Check sheet for the modelled part. Datum: model origin and axes. Units: mm. Coordinates: 2 decimals unless noted, no trailing zeros. Order: outer loops, then holes, each group sorted by start corner. A loop starts at its lowest first (then second) coordinate and runs counter-clockwise, first axis right, second up.
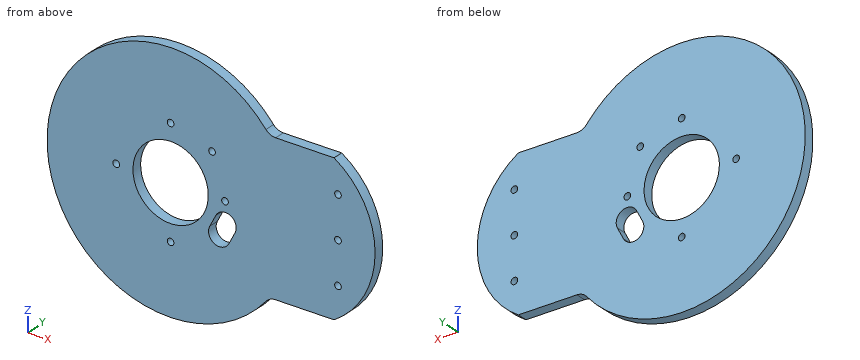
from build123d import *

# Parameters (mm, degrees)
SKETCH1_R                   = 2.0193
BOSS_EXTRUDE1_DEPTH         = 6.35
SKETCH16_R                  = 22.86
SKETCH16_R_2                = 2.0193
CUT_EXTRUDE1_DEPTH          = 6.35
FILLET1_R                   = 7.62
F_21_0_159_DIAMETER_HOLE1_D = 4.0386
CUT_EXTRUDE2_DEPTH          = 168.826775285
CUT_EXTRUDE3_DEPTH          = 168.826775285


with BuildPart() as part:
    # Sketch1 → Boss-Extrude1 (new body)
    with BuildSketch(Plane(origin=(0, 0, 0), x_dir=(1, 0, 0), z_dir=(0, 1, 0))):
        with BuildLine():
            Line((24.199172761, -44.999955873), (-14.950739381, -44.936113543))
            ThreePointArc((-14.950739381, -44.936113543), (-150.001077441, -0.07990002), (-15.0466181, 45.063954554))
            Line((-15.0466181, 45.063954554), (24.199172761, 44.999955873))
            ThreePointArc((24.199172761, 44.999955873), (71.663954553, 0), (24.199172761, -44.999955873))
        make_face()
        with Locations(Location((26.6, 0, 0), (0, 0, 270))):
            Circle(SKETCH1_R, mode=Mode.SUBTRACT)
    extrude(amount=BOSS_EXTRUDE1_DEPTH)

    # Sketch16 → Cut-Extrude1 (cut)
    with BuildSketch(Plane(origin=(0.964771866, 6.35, 105.934324836), x_dir=(-1, 0, 0), z_dir=(0, 1, 0))):
        with Locations(Location((75.964771866, -105.934324836, 0), (0, 0, 90))):
            Circle(SKETCH16_R)
        with Locations(Location((50.800979112, -80.770532082, 0), (0, 0, 90))):
            Circle(SKETCH16_R_2)
        with Locations(Location((42.944771866, -105.934324836, 0), (0, 0, 90))):
            Circle(SKETCH16_R_2)
        with Locations(Location((75.964771866, -72.914324836, 0), (0, 0, 90))):
            Circle(SKETCH16_R_2)
        with Locations(Location((108.984771866, -105.934324836, 0), (0, 0, 90))):
            Circle(SKETCH16_R_2)
        with Locations(Location((75.964771866, -138.954324836, 0), (0, 0, 90))):
            Circle(SKETCH16_R_2)
    extrude(amount=-CUT_EXTRUDE1_DEPTH, mode=Mode.SUBTRACT)

    # Fillet1
    fillet1_edges = [part.edges().sort_by_distance(p)[0] for p in [
        (-15.0466181, 3.175, -45.063954554),
        (-14.950739381, 3.175, 44.936113543),
    ]]
    fillet(fillet1_edges, radius=FILLET1_R)

    # #21 (0.159) Diameter Hole1 (through all)
    with Locations(Plane(origin=(0, 6.35, 0), x_dir=(1, 0, 0), z_dir=(0, 1, 0))):
        with Locations((26.6, 25.4), (26.6, -25.4)):
            Hole(F_21_0_159_DIAMETER_HOLE1_D / 2)

    # Sketch19 → Cut-Extrude2 (cut, through all)
    with BuildSketch(Plane(origin=(0, 6.35, 0), x_dir=(1, 0, 0), z_dir=(0, 1, 0))):
        with BuildLine():
            ThreePointArc((24.199172761, 44.999955873), (49.131977277, 0), (24.199172761, -44.999955873))
            ThreePointArc((24.199172761, -44.999955873), (71.663954553, 0), (24.199172761, 44.999955873))
        make_face()
    extrude(amount=-CUT_EXTRUDE2_DEPTH, mode=Mode.SUBTRACT)

    # Sketch20 → Cut-Extrude3 (cut, through all)
    with BuildSketch(Plane(origin=(0, 6.35, 0), x_dir=(1, 0, 0), z_dir=(0, 1, 0))):
        with BuildLine():
            Line((-39.61253295, 22.813806704), (-35.939374007, 15.716554888))
            ThreePointArc((-35.939374007, 15.716554888), (-38.746700574, 6.886169325), (-47.577086137, 9.693495892))
            Line((-47.577086137, 9.693495892), (-51.25024508, 16.790747709))
            ThreePointArc((-51.25024508, 16.790747709), (-48.442918513, 25.621133271), (-39.61253295, 22.813806704))
        make_face()
    extrude(amount=-CUT_EXTRUDE3_DEPTH, mode=Mode.SUBTRACT)


solid = part.part
(1) Cross-section at B-B (x = -75). Enter the section's corners in (y, z), and give its area (3 significant figures).
Filled in:
outline: (0, -75) - (6.35, -75) - (6.35, -35.04) - (0, -35.04) - close; (0, -31) - (6.35, -31) - (6.35, -22.86) - (0, -22.86) - close; (0, 22.86) - (6.35, 22.86) - (6.35, 31) - (0, 31) - close; (0, 35.04) - (6.35, 35.04) - (6.35, 75) - (0, 75) - close
area: 611 mm2
(2) Cross-section at C-C (y = 5). Count the separate pieces of the cut face and the enclosed holes in it, and give its area (3 significant figures).
Filled in:
separate pieces: 1
enclosed holes: 10
area: 19,900 mm2
(3) Go/stop test with flat-tipped pins: P1, Ø3, axis at x = -75, z = -33.02, coming from the -Y side; P2, Ø1.5, axis at x = 29, y = 3.5, coming from the +Z side; P3, Ø1.5, axis at x = -77, y = 4.5, coming from the +Z side. Record where each tip stops, or that it passes through.
Filled in:
P1: passes through
P2: stops at z = 42.2
P3: stops at z = 74.99
(4) Cross-section at A-A (z = 0). Enter the section's corners in (x, y).
Filled in:
outline: (-150, 0) - (-110.04, 0) - (-110.04, 6.35) - (-150, 6.35) - close; (-106, 0) - (-97.86, 0) - (-97.86, 6.35) - (-106, 6.35) - close; (-52.14, 0) - (-44, 0) - (-44, 6.35) - (-52.14, 6.35) - close; (-39.96, 0) - (24.58, 0) - (24.58, 6.35) - (-39.96, 6.35) - close; (28.62, 0) - (49.13, 0) - (49.13, 6.35) - (28.62, 6.35) - close
(5) Cross-section at D-D (z = -33.02). Enter the section's corners in (x, y), and give its area (3 significant figures).
Filled in:
outline: (-142.34, 0) - (-77.02, 0) - (-77.02, 6.35) - (-142.34, 6.35) - close; (-72.98, 0) - (37.61, 0) - (37.61, 6.35) - (-72.98, 6.35) - close
area: 1,120 mm2
(6) Thickness scan on probe 1 along X at (y, z) = (2, 0); probe 2 along X at (y, z) = (2.5, 25.4); probe 3 along Z at (x, y) = (4.5, 2.5). Record the ranges inside material, lowest first.
Filled in:
probe 1: x = -150 to -110.04, -106 to -97.86, -52.14 to -44, -39.96 to 24.58, 28.62 to 49.13
probe 2: x = -145.57 to -51.84, -47.83 to 24.58, 28.62 to 42.66
probe 3: z = -45.03 to 44.97
